Design review of the part shown in the three views and the two pictorial views. Dimensions are in mm from the part's minimum x, y and z. A direction names the side the tool comes from. Give positions to 0.01 mm unless a question says otherwise; leave off trailing zeros. Write each loop counter-clockwise with the first axis right and the second up, starting at its lowest first coordinate (ties: lowest second). Pieces come first, ordered by that corner, then holes. Notation, with made-up numbers: M 72,20 L 106,20 A11 ccw 106,35 Z; hole C 70,13.25 d9. An arc over 180 degrees is marked long. Use one line per item in the form item = value. Start each with the question number.
Q1. Tool access review of the marked faces 4, 5, 6 and 7: name each direction out of +Z, -Z, +X, -X, +Y, -Y from which nothing blocks a thin tool from reaching the whole face with its end or side.
Q2. Mouldability with a two-part tool opening along Z and no side actions: class the marked faces 1, 2 and 3 as released by +Z, released by -Z, zero draft, split by the parting line, or undercut.
Q3. Consider section A-A on y = 3. Write out the cut boundary in (x, z).
Q4. For probe 1 along Y at (x, z) = (8, 4.75); probe 2 along X at (y, z) = (3, 3.6); probe 3 along Z at (x, y) = (9.25, 3.75), list the stretches that pass through material, from the lowest coordinate up. Write a range as [from, to].
Q5. Consider section D-D on y = 1.15. Write out the cut boundary in (x, z).
Q6. Consider section C-C on x = 8.5. Write out the cut boundary in (y, z).
Q7. Clearance check with flat-ended pins moving along their axes: pin 1 Ø2 at (y, z) = (2, 3.5) entering from +X; pin 2 Ø4 at (x, z) = (9, 6.5) entering from -Y; pin 3 Ø4 at (x, z) = (5.5, 3) entering from +Y. State where each tip first meets the part, or that it passes through.
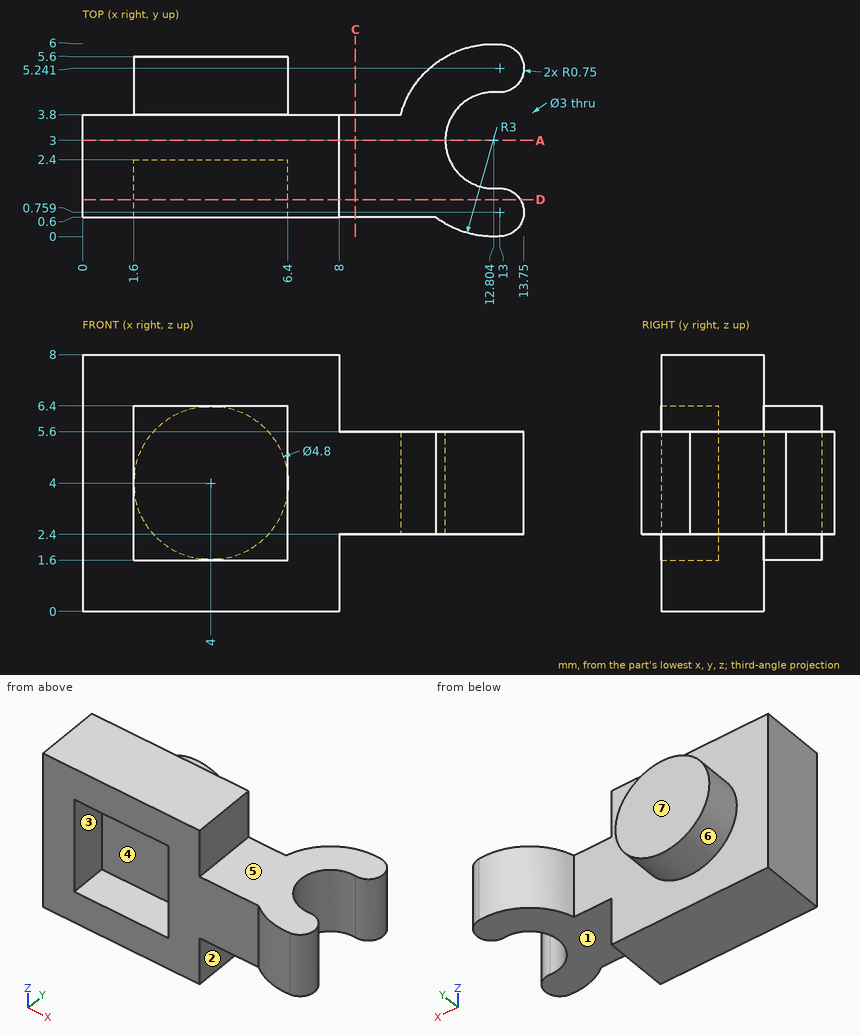
Working result:
q1.face_4 = -Y
q1.face_5 = +Z, +X, +Y, -Y
q1.face_6 = +Y
q1.face_7 = +Z, -Z, -X, +Y
q2.face_1 = released by -Z
q2.face_2 = zero draft
q2.face_3 = undercut
q3.outline = M 0,0 L 8,0 L 8,2.4 L 11.3,2.4 L 11.3,5.6 L 8,5.6 L 8,8 L 0,8 Z
q4.probe_1 = [0.6, 3.8]
q4.probe_2 = [0, 11.3]
q4.probe_3 = [2.4, 5.6]
q5.outline = M 0,0 L 8,0 L 8,2.4 L 13.64,2.4 L 13.64,5.6 L 8,5.6 L 8,8 L 0,8 Z; hole M 1.6,1.6 L 6.4,1.6 L 6.4,6.4 L 1.6,6.4 Z
q6.outline = M 0.6,2.4 L 3.8,2.4 L 3.8,5.6 L 0.6,5.6 Z
q7.pin_1 = 13.71
q7.pin_2 = 0.6
q7.pin_3 = 5.6
